Here's how the part is built. I have some questions about the finished solid (model axes, mm). A direction names the side the tool comes from. Round coordinates to 2 decimals unless told otherwise and drop trailing zeros. Order: outer loops, then holes, each group sorted by start corner. A loop starts at its lowest first (then second) coordinate and runs counter-clockwise, first axis right, second up. Notation, with made-up numbers: (5.25, -15.75) - (62.25, -15.75) arc R20 cw to (62.25, 20.25) - close; hole circle Ø8 at (7, 3.5). An arc over 180 degrees is marked (long way). Answer as a JSON object with one key per item and string values.
```python
from build123d import *

# Parameters (mm, degrees)
F1_DEPTH      = 644
F2_R          = 5
F2_R_2        = 2
F3_DEPTH      = 40
F8_W          = 94.9183702469
F8_H          = 83.3485722542
F9_DEPTH      = 11
F9_DEPTH_BACK = 25


with BuildPart() as f1:
    # F0 (on Top) → F1 (new body)
    with BuildSketch(Plane.XY):
        with BuildLine():
            Line((15, 15), (-15, 15))
            ThreePointArc((-15, 15), (-25.6066017178, 10.6066017178), (-30, 0))
            ThreePointArc((-30, 0), (-25.6066017178, -10.6066017178), (-15, -15))
            Line((-15, -15), (15, -15))
            ThreePointArc((15, -15), (25.6066017178, -10.6066017178), (30, 0))
            ThreePointArc((30, 0), (25.6066017178, 10.6066017178), (15, 15))
        make_face()
        with BuildLine():
            ThreePointArc((-28.5, 0), (-24.545941546, 9.545941546), (-15, 13.5))
            Line((-15, 13.5), (15, 13.5))
            ThreePointArc((15, 13.5), (24.545941546, 9.545941546), (28.5, 0))
            ThreePointArc((28.5, 0), (24.545941546, -9.545941546), (15, -13.5))
            Line((15, -13.5), (-15, -13.5))
            ThreePointArc((-15, -13.5), (-24.545941546, -9.545941546), (-28.5, 0))
        make_face(mode=Mode.SUBTRACT)
    extrude(amount=-F1_DEPTH)

    # F2 (on face) → F3 (cut)
    with BuildSketch(Plane(origin=(0, 15, 0), x_dir=(-1, 0, 0), z_dir=(0, 1, 0))):
        with Locations((0, -15)):
            Circle(F2_R)
        with Locations((0, -39)):
            Circle(F2_R_2)
    extrude(amount=-F3_DEPTH, mode=Mode.SUBTRACT)

    # F8 (on face) → F9 (cut, two sides)
    with BuildSketch(Plane(origin=(-194.0232580496, 182.3222238501, -500.9261930928), x_dir=(0.9396926208, 0.1169777784, -0.3213938048), z_dir=(-0.3420201433, 0.3213938048, -0.8830222216))) as f9_sk:
        with Locations((206.5364569426, 219.5619344711)):
            Rectangle(F8_W, F8_H)
    extrude(amount=-F9_DEPTH, mode=Mode.SUBTRACT)
    extrude(f9_sk.sketch, amount=F9_DEPTH_BACK, mode=Mode.SUBTRACT)


solid = f1.part
```
1. Thinking about a two-plate mould opening in Z: for faces 3 (the face through (-0.14, 13.741, -624.924)), 4 (the face through (1.08, 14.26, -19.88)), 5 (the face through (0, 15, -311)), which applies, pulls with the +Z half, pulls with the -Z half, needs draft (parallel to the pull), parting line crosses it, or undercut?
Responses:
{"face 3": "pulls with the -Z half", "face 4": "undercut", "face 5": "needs draft"}
2. For P1, Ø1, axis at x = -17, z = -490.5, coming from the -Y side; P2, Ø5, axis at y = 3, z = -396, coming from the -X side; P3, Ø8, axis at y = 7.5, z = -157, coming from the +X side, each with a flat end and sliding along its axis, tell me the tip position at first contact or that it passes through.
Responses:
{"P1": "y = -14.92", "P2": "x = -29.99", "P3": "x = 29.59"}
3. Imagine slicing it at B-B (y = -9). List the corners of the cut face in (x, z) for me, plus the area to 3 significant figures.
Responses:
{"outline": "(-27, -622.8) - (-25.06, -623.55) - (-25.06, 0) - (-27, 0) - close; (25.06, -642.96) - (27, -643.71) - (27, 0) - (25.06, 0) - close", "area": "2,450 mm2"}
4. Imagine slicing it at A-A (z = -72). List the corners of the cut face in (x, y) for me, plus the area to 3 significant figures.
Responses:
{"outline": "(-15, -15) - (15, -15) arc R15 ccw to (15, 15) - (-15, 15) arc R15 ccw to start; hole (-15, -13.5) - (15, -13.5) arc R13.5 ccw to (15, 13.5) - (-15, 13.5) arc R13.5 ccw to start", "area": "224 mm2"}
5. For faces 1 (the face through (0, -13.5, -316)), 2 (the face through (-30, 0, -310)), which set-ups out of +Z, -Z, +X, -X, +Y, -Y let a thin tool reach every point of the face, with its end or its side?
Responses:
{"face 1": "+Z, -Z", "face 2": "+Z, -Z, -X"}
6. If I drill on L1, parallel to Y at x = 14, z = -264; L2, parallel to X at y = 1, z = -122; L3, parallel to Z at x = 0, y = 14.1, over which ranges is the centre line in solid material (lowest first)? Write a range as [from, to].
Responses:
{"L1": "[-15, -13.5], [13.5, 15]", "L2": "[-29.97, -28.46], [28.46, 29.97]", "L3": "[-624.85, -41], [-37, -20], [-10, 0]"}
